Here's how the part is built. I have some questions about the finished solid (model axes, mm). Face numbers are marked on the shaded views. A direction names the side the tool comes from. Round coordinates to 2 decimals unless told otherwise and drop trailing zeros. Order: outer loops, then holes, each group sorted by start corner. A loop starts at its lowest first (then second) coordinate and runs counter-clockwise, first axis right, second up. Notation, with made-up numbers: (-34.5, 42) -> (13.5, 42) arc R20 cw to (13.5, 48) -> close; hole circle Ø4 at (72, 27). An arc over 180 degrees is marked (long way). Use a Markdown table: item, result. Add a question column.
from build123d import *

# Parameters (mm, degrees)
SKETCH1_R           = 1.7
BOSS_EXTRUDE1_DEPTH = 5
FILLET1_R           = 3
SKETCH2_W           = 82.534528382
SKETCH2_H           = 8
BOSS_EXTRUDE2_DEPTH = 6
FILLET2_R           = 4
SKETCH3_W           = 22
SKETCH3_H           = 9
BOSS_EXTRUDE3_DEPTH = 4
FILLET3_R           = 3
SKETCH4_R           = 1.7
CUT_EXTRUDE2_DEPTH  = 4
FILLET4_R           = 3
FILLET5_R           = 3


with BuildPart() as part:
    # Sketch1 → Boss-Extrude1 (new body)
    with BuildSketch(Plane(origin=(0, 0, 0), x_dir=(1, 0, 0), z_dir=(0, 1, 0))):
        Polygon((-76.5, -12), (-53.5, -12), (53.5, -12), (76.5, -12), (76.5, 12), (53.5, 12), (-53.5, 12), (-76.5, 12), align=None)
        with Locations(Location((-72.5, 8, 0), (0, 0, 270))):
            Circle(SKETCH1_R, mode=Mode.SUBTRACT)
        with Locations(Location((-57.5, 8, 0), (0, 0, 270))):
            Circle(SKETCH1_R, mode=Mode.SUBTRACT)
        with Locations(Location((-57.5, -8, 0), (0, 0, 270))):
            Circle(SKETCH1_R, mode=Mode.SUBTRACT)
        with Locations(Location((-72.5, -8, 0), (0, 0, 270))):
            Circle(SKETCH1_R, mode=Mode.SUBTRACT)
        with Locations(Location((57.5, 8, 0), (0, 0, 270))):
            Circle(SKETCH1_R, mode=Mode.SUBTRACT)
        with Locations(Location((72.5, 8, 0), (0, 0, 270))):
            Circle(SKETCH1_R, mode=Mode.SUBTRACT)
        with Locations(Location((72.5, -8, 0), (0, 0, 270))):
            Circle(SKETCH1_R, mode=Mode.SUBTRACT)
        with Locations(Location((57.5, -8, 0), (0, 0, 270))):
            Circle(SKETCH1_R, mode=Mode.SUBTRACT)
    extrude(amount=BOSS_EXTRUDE1_DEPTH)

    # Fillet1
    fillet1_edges = [part.edges().sort_by_distance(p)[0] for p in [
        (-76.5, 2.5, 12),
        (-76.5, 2.5, -12),
        (76.5, 2.5, -12),
        (76.5, 2.5, 12),
    ]]
    fillet(fillet1_edges, radius=FILLET1_R)

    # Sketch2 → Boss-Extrude2 (add)
    with BuildSketch(Plane(origin=(0, 5, 0), x_dir=(1, 0, 0), z_dir=(0, 1, 0))):
        with Locations((0, -2.722781506)):
            Rectangle(SKETCH2_W, SKETCH2_H)
    extrude(amount=BOSS_EXTRUDE2_DEPTH)

    # Fillet2
    fillet2_edges = [part.edges().sort_by_distance(p)[0] for p in [
        (0, 11, 6.722781506),
        (0, 11, -1.277218494),
    ]]
    fillet(fillet2_edges, radius=FILLET2_R - 0.0001)  # a hair under: the kernel refuses the full size

    # Sketch3 → Boss-Extrude3 (add)
    with BuildSketch(Plane(origin=(0, 0, -12), x_dir=(-1, 0, 0), z_dir=(0, 0, -1))):
        with Locations((-11, 9.5)):
            Rectangle(SKETCH3_W, SKETCH3_H)
        with Locations((11, 9.5)):
            Rectangle(SKETCH3_W, SKETCH3_H)
    extrude(amount=-BOSS_EXTRUDE3_DEPTH)

    # Fillet3
    fillet3_edges = [part.edges().sort_by_distance(p)[0] for p in [
        (-22, 5, -10),
        (22, 5, -10),
    ]]
    fillet(fillet3_edges, radius=FILLET3_R)

    # Sketch4 → Cut-Extrude2 (cut)
    with BuildSketch(Plane(origin=(0, 0, -12), x_dir=(-1, 0, 0), z_dir=(0, 0, -1))):
        with BuildLine():
            ThreePointArc((-15.3, 10), (-15.797918472, 11.202081528), (-17, 11.7))
            Line((-17, 11.7), (-17, 10))
            Line((-17, 10), (-18.7, 10))
            ThreePointArc((-18.7, 10), (-17, 8.3), (-15.3, 10))
        make_face()
        with BuildLine():
            Line((-17, 10), (-17, 11.7))
            ThreePointArc((-17, 11.7), (-18.202081528, 11.202081528), (-18.7, 10))
            Line((-18.7, 10), (-17, 10))
        make_face()
        with Locations((17, 10)):
            Circle(SKETCH4_R)
    extrude(amount=-CUT_EXTRUDE2_DEPTH, mode=Mode.SUBTRACT)

    # Fillet4
    fillet4_edges = [part.edges().sort_by_distance(p)[0] for p in [
        (22, 14, -10),
        (-22, 14, -10),
    ]]
    fillet(fillet4_edges, radius=FILLET4_R)

    # Fillet5
    fillet5_edges = [part.edges().sort_by_distance(p)[0] for p in [
        (0, 5, -8),
    ]]
    fillet(fillet5_edges, radius=FILLET5_R)


solid = part.part
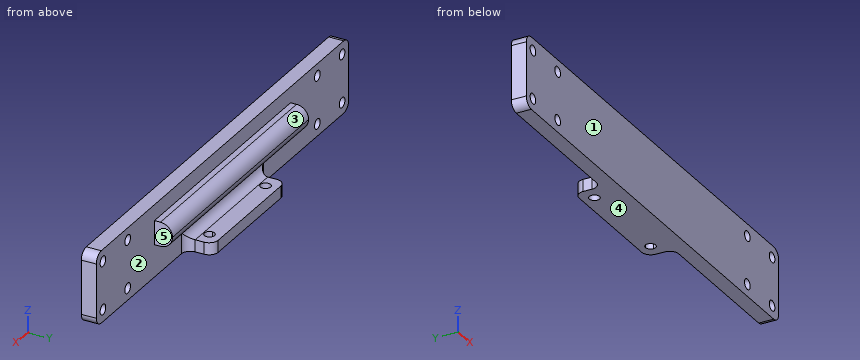
(1) If we mould it in two halves opening along Z, with no side actions, what happens to the marked faces 3, 4 and 5? For each: pulls with the +Z half, pulls with the -Z half, needs draft (parallel to the pull), parting line crosses it, or undercut.
(2) I want a section at C-C on z = 4.5. List the corners of the cut face in (x, y) for me.
(3) I'm going to push flat-ended pins straight in: P1, Ø1.5, axis at x = 35.5, y = 9.5, coming from the +Z side; P2, Ø4, axis at x = 72.5, z = 8, coming from the -Y side; P3, Ø2, axis at x = 58, z = -1, coming from the +Y side; P4, Ø4, axis at x = -17, y = 10, coming from the +Z side. Where does each tip first touch, or does it pass through?
(4) On a 3-axis mill with a long thin cutter (end or side, diameter ignored), from which of +Z, -Z, +X, -X, +Y, -Y can I reach the whole of each face in a straight line? I mean the marked faces 1 and 2. Say none if no direction works.
(5) I want a section at A-A on x = 57.5. List the corners of the cut face in (y, z) for me.
(6) I want a section at B-B on y = 2.25. State how many separate pieces and enclosed holes the cut face has, and give its area (3 significant figures).
(7) Please list where these lines run through material, in increasing order: probe 1 along X at (y, z) = (3.9, -8); probe 2 along Z at (x, y) = (-72.5, 1.85); probe 3 along Y at (x, z) = (-31.5, 2.5). Write a range as from..to.
Output:
| question | item | result |
|---|---|---|
| 1 | face 3 | pulls with the +Z half |
| 1 | face 4 | pulls with the -Z half |
| 1 | face 5 | needs draft |
| 2 | outline | (-76.5, 0) -> (76.5, 0) -> (76.5, 5) -> (41.27, 5) -> (41.27, 10.58) -> (-41.27, 10.58) -> (-41.27, 5) -> (-76.5, 5) -> close |
| 3 | P1 | z = 6.32 |
| 3 | P2 | y = 0 |
| 3 | P3 | y = 5 |
| 3 | P4 | z = 6.6 |
| 4 | face 1 | +Z, -Z, +X, -X, -Y |
| 4 | face 2 | +Y |
| 5 | outline | (0, -12) -> (5, -12) -> (5, -9.7) -> (0, -9.7) -> close; (0, -6.3) -> (5, -6.3) -> (5, 6.3) -> (0, 6.3) -> close; (0, 9.7) -> (5, 9.7) -> (5, 12) -> (0, 12) -> close |
| 6 | separate pieces | 1 |
| 6 | enclosed holes | 8 |
| 6 | area | 3,590 mm² |
| 7 | probe 1 | -76.5..-74.2, -70.8..-59.2, -55.8..55.8, 59.2..70.8, 74.2..76.5 |
| 7 | probe 2 | -12..-9.7, -6.3..6.3, 9.7..12 |
| 7 | probe 3 | 0..10.99 |
